The listing builds one solid part. Answer for the finished solid, in the listing's coordinates (mm). A direction names the side the tool comes from. Coordinates: 2 decimals unless noted, no trailing zeros. Order: outer loops, then holes, each group sorted by start corner. A loop starts at its lowest first (then second) coordinate and runs counter-clockwise, first axis right, second up.
from build123d import *

# Parameters (mm, degrees)
F0_R          = 3.25
F0_R_2        = 2.125
F0_R_3        = 4.25
F1_DEPTH      = 5
F2_W          = 25
F2_H          = 5
F3_DEPTH      = 25
F4_R          = 7.25
F4_R_2        = 3.25
F4_R_3        = 8.25
F4_R_4        = 4.25
F5_DEPTH      = 10
F6_R          = 2.125
F7_DEPTH      = 5.001
F8_W          = 5
F8_H          = 17.15
F8_W_2        = 4
F8_H_2        = 13.3875096302
F9_DEPTH      = 10
F10_T1_DEPTH  = 5
F10_T3_DEPTH  = 4
F10_T8_DEPTH  = 30.7168298797
F10_T13_DEPTH = 29.7168298797
F10_T18_DEPTH = 27.1526880508
F10_S20_R     = 3.25
F10_T21_DEPTH = 16
F10_T25_DEPTH = 13.3875096302


# Not quite as in the source:
# - a fillet or chamfer that OpenCascade refuses, or shapes differently, is made with other operations: its cross-section is extruded or revolved along the edge and cut away or added


with BuildPart() as f1:
    # F0 (on Top) → F1 (new body)
    with BuildSketch(Plane.XY):
        with BuildLine():
            Line((12.5, 26.5), (0, 26.5))
            Line((0, 26.5), (-12.5, 26.5))
            Line((-12.5, 26.5), (-12.5, 7.0478720193))
            ThreePointArc((-12.5, 7.0478720193), (-17.9845104515, -0.9722703187), (-10.5656007648, -7.2462098368))
            Line((-10.5656007648, -7.2462098368), (-7.5, -7.2462098368))
            Line((-7.5, -7.2462098368), (-7.5, -13.6))
            ThreePointArc((-7.5, -13.6), (-5.3033008589, -18.9033008589), (0, -21.1))
            ThreePointArc((0, -21.1), (5.3033008589, -18.9033008589), (7.5, -13.6))
            Line((7.5, -13.6), (7.5, -8.25))
            ThreePointArc((7.5, -8.25), (15.3166703137, -2.6385915194), (12.5, 6.5622023742))
            Line((12.5, 6.5622023742), (12.5, 26.5))
        make_face()
        with Locations((-10.8, 0)):
            Circle(F0_R, mode=Mode.SUBTRACT)
        with Locations((0, -13.6)):
            Circle(F0_R_2, mode=Mode.SUBTRACT)
        with Locations((7.5, 0)):
            Circle(F0_R_3, mode=Mode.SUBTRACT)
        with Locations((0, 16.5)):
            Circle(F0_R_2, mode=Mode.SUBTRACT)
    extrude(amount=F1_DEPTH)

    # F2 (on face) → F3 (join)
    with BuildSketch(Plane.XY.offset(5)):
        with Locations((0, 24)):
            Rectangle(F2_W, F2_H)
    extrude(amount=F3_DEPTH)

    # F4 (on face) → F5 (join)
    with BuildSketch(Plane.XY.offset(5)):
        with Locations((-10.8, 0)):
            Circle(F4_R)
        with Locations((-10.8, 0)):
            Circle(F4_R_2, mode=Mode.SUBTRACT)
        with Locations((7.5, 0)):
            Circle(F4_R_3)
        with Locations((7.5, 0)):
            Circle(F4_R_4, mode=Mode.SUBTRACT)
    extrude(amount=F5_DEPTH)

    # F6 (on face) → F7 (cut, through all)
    with BuildSketch(Plane.XZ.offset(-21.5)):
        with Locations((0, 22.5)):
            Circle(F6_R)
    extrude(amount=-F7_DEPTH, mode=Mode.SUBTRACT)

    # F8 (on face) → F9 (join)
    with BuildSketch(Plane.XY.offset(5)):
        with Locations((-7.5, 12.925)):
            Rectangle(F8_W, F8_H)
        with Locations((8, 14.8062451849)):
            Rectangle(F8_W_2, F8_H_2)
    extrude(amount=F9_DEPTH)

    # F10: chamfer of 5 on 4 edges, made by hand

    # F10_s2 → F10_t1 (join)
    with BuildSketch(Plane.YZ.offset(-10)):
        Polygon((16.5, 15), (21.5, 20), (21.5, 15), align=None)
    extrude(amount=F10_T1_DEPTH)

    # F10_s4 → F10_t3 (join)
    with BuildSketch(Plane.YZ.offset(6)):
        Polygon((21.5, 20), (16.5, 15), (21.5, 15), align=None)
    extrude(amount=F10_T3_DEPTH)


with BuildPart() as f10_tool6:
    # F10_s7 → F10_t8 (new body)
    with BuildSketch(Plane.YZ.offset(7.8584149398)):
        Polygon((16.5, 15), (21.5, 20), (21.5, 15), align=None)
    extrude(amount=-F10_T8_DEPTH)

    split(bisect_by=Plane.YZ.offset(6), keep=Keep.TOP)


with BuildPart() as f1_1:
    add(f1.part)

    # F10_t5: union F10_tool6
    add(f10_tool6.part)


with BuildPart() as f10_tool11:
    # F10_s12 → F10_t13 (new body)
    with BuildSketch(Plane.YZ.offset(22.8584149398)):
        Polygon((21.5, 20), (16.5, 15), (21.5, 15), align=None)
    extrude(amount=-F10_T13_DEPTH)

    split(bisect_by=Plane.YZ.offset(-5), keep=Keep.BOTTOM)


with BuildPart() as f1_2:
    add(f1_1.part)

    # F10_t10: union F10_tool11
    add(f10_tool11.part)


with BuildPart() as f10_tool16:
    # F10_s17 → F10_t18 (new body)
    with BuildSketch(Plane.XZ.offset(-21.5)):
        Polygon((-10, 10), (-15, 5), (-10, 5), align=None)
    extrude(amount=F10_T18_DEPTH)

    split(bisect_by=Plane.YZ.offset(-12.5), keep=Keep.TOP)

    # F10_s20 → F10_t21 (cut, symmetric)
    with BuildSketch(Plane.XY.offset(7.5)):
        with Locations((-10.8, 0)):
            Circle(F10_S20_R)
    extrude(amount=F10_T21_DEPTH, both=True, mode=Mode.SUBTRACT)


with BuildPart() as f1_3:
    add(f1_2.part)

    # F10_t15: union F10_tool16
    add(f10_tool16.part)


with BuildPart() as f10_tool23:
    # F10_s24 → F10_t25 (new body)
    with BuildSketch(Plane.XZ.offset(-8.1124903698)):
        Polygon((10, 10), (15, 5), (10, 5), align=None)
    extrude(amount=-F10_T25_DEPTH)

    split(bisect_by=Plane.YZ.offset(12.5), keep=Keep.BOTTOM)


with BuildPart() as f1_4:
    add(f1_3.part)

    # F10_t22: union F10_tool23
    add(f10_tool23.part)


solid = f1_4.part
(1) Given pin 1 Ø0.8 at (x, y) = (10.5, 7.5) entering from +Z; pin 2 Ø2.5 at (y, z) = (-11.5, 1.5) entering from -X; pin 3 Ø1 at (y, z) = (3, 5) entering from +X, each flat-ended and moving along its own axis, determine where each tip first touches the part or whether it passes through.
(2) The mould has two halves that part along Z. Classify faces 6 (the flat face through (11, 15, 9)), 7 (the cylindrical face through (-0.461, 23.965, 20.426)), 8 (the cylindrical face through (2.027, 17.138, 2.465)): pulls with the +Z half, pulls with the -Z half, needs draft (parallel to the pull), parting line crosses it, or undercut.
(3) Find section A-A on z = 22.5. Determine the outline of the cut face in (x, y) (3 decimals), then the cut area to 3 significant figures.
(4) Find section C-C on x = -6.5. Determine the outline of the cut face in (y, z).
(5) A tool of negligible diameter and unlimited length cuts with its end or side. For faces 1 (the flat face through (-12.5, 23, 9)), 2 (the flat face through (12.5, 23, 12)), 3 (the flat face through (10, 16, 13)), 4 (the flat face through (-7.5, -10, 2)), 5 (the flat face through (6, 15, 11)), from which of +Z, -Z, +X, -X, +Y, -Y can it reach the whole face along a straight path? Write none if from no direction.
(6) Find the intervals of material crossed by probe 1 along Y at (x, z) = (-11, 12.25); probe 2 along Y at (x, z) = (0, 3.75) (3 decimals); probe 3 along Y at (x, z) = (-10.8, 4), in increasing order.
(7) Find section D-D on z = 16. Determine the outline of the cut face in (x, y), then the cut area to 3 significant figures.
(8) Find section B-B on y = 0. Determine the outline of the cut face in (x, z).
Resolved:
1. pin 1: stops at z = 15
1. pin 2: stops at x = -7.5
1. pin 3: stops at x = 15.36
2. face 6: pulls with the +Z half
2. face 7: undercut
2. face 8: needs draft
3. outline: (-12.5, 21.5) - (-2.125, 21.5) - (-2.125, 26.5) - (-12.5, 26.5) - close; (2.125, 21.5) - (12.5, 21.5) - (12.5, 26.5) - (2.125, 26.5) - close
3. area: 104 mm2
4. outline: (-17.34, 0) - (26.5, 0) - (26.5, 30) - (21.5, 30) - (21.5, 20) - (16.5, 15) - (-5.84, 15) - (-5.84, 5) - (-17.34, 5) - close
5. face 1: +Z, -Z, -X, +Y
5. face 2: +Z, -Z, +X, +Y
5. face 3: +Z, +X
5. face 4: +Z, -Z, -X, -Y
5. face 5: +Z
6. probe 1: y = -7.25 to -3.24, 3.24 to 7.25, 21.5 to 26.5
6. probe 2: y = -21.1 to -15.725, -11.475 to 14.375, 18.625 to 26.5
6. probe 3: y = -7.25 to -3.25, 3.25 to 26.5
7. outline: (-12.5, 21.5) - (-10, 21.5) - (-10, 17.5) - (-5, 17.5) - (-5, 21.5) - (6, 21.5) - (6, 17.5) - (10, 17.5) - (10, 21.5) - (12.5, 21.5) - (12.5, 26.5) - (-12.5, 26.5) - close
7. area: 161 mm2
8. outline: (-18.05, 0) - (-14.05, 0) - (-14.05, 15) - (-18.05, 15) - close; (-7.55, 0) - (3.25, 0) - (3.25, 15) - (-0.75, 15) - (-0.75, 5) - (-3.55, 5) - (-3.55, 15) - (-7.55, 15) - close; (11.75, 0) - (15.75, 0) - (15.75, 15) - (11.75, 15) - close
